from build123d import *

# Parameters (mm, degrees)
SKETCH1_W           = 16
SKETCH1_H           = 9
BOSS_EXTRUDE1_DEPTH = 3


with BuildPart() as part:
    # Sketch1 → Boss-Extrude1 (new body)
    with BuildSketch(Plane(origin=(0, 0, 0), x_dir=(0, 0, -1), z_dir=(1, 0, 0))):
        Polygon((10, 153.005875518), (20, 153.005875518), (20, 150.005875518), (30, 150.005875518), (30, 153.005875518), (40, 153.005875518), (40, 150.005875518), (50, 150.005875518), (50, 153.005875518), (60, 153.005875518), (60, 150.005875518), (70, 150.005875518), (70, 140), (73, 140), (73, 130), (70, 130), (70, 120), (73, 120), (73, 110), (70, 110), (70, 100), (73, 100), (73, 90), (70, 90), (70, 80), (73, 80), (73, 70), (70, 70), (70, 60), (73, 60), (73, 50), (70, 50), (70, 40), (73, 40), (73, 30), (70, 30), (70, 20), (73, 20), (73, 10), (70, 10), (70, 0), (60, 0), (60, -3), (50, -3), (50, 0), (40, 0), (40, -3), (30, -3), (30, 0), (20, 0), (20, -3), (10, -3), (10, 0), (0, 0), (0, 10), (-3, 10), (-3, 20), (0, 20), (0, 30), (-3, 30), (-3, 40), (0, 40), (0, 50), (-3, 50), (-3, 60), (0, 60), (0, 70), (-3, 70), (-3, 80), (0, 80), (0, 90), (-3, 90), (-3, 100), (0, 100), (0, 110), (-3, 110), (-3, 120), (0, 120), (0, 130), (-3, 130), (-3, 140), (0, 140), (0, 150.005875518), (10, 150.005875518), align=None)
        with Locations((33.90899457, 144.39356925)):
            Rectangle(SKETCH1_W, SKETCH1_H, mode=Mode.SUBTRACT)
    extrude(amount=BOSS_EXTRUDE1_DEPTH)


solid = part.part
Check sheet for the modelled part. Datum: model origin and axes. Units: mm. A direction names the side the tool comes from. Round coordinates to 2 decimals unless told otherwise and drop trailing zeros. Loops run counter-clockwise (first coordinate to the right, second up) from the corner with the lowest first, then second, coordinate; pieces in that order, holes last.
1. Sectioned sample at C-C on z = -62. Record the boundary of the cut face in (x, y).
2. Set-up check for faces 5 (the flat face through (1, 139.894, -34)), 6 (the flat face through (1, 140, 2)), 7 (the flat face through (1, 130, 1)), 8 (the flat face through (1, 150.006, -45)), 9 (the flat face through (1, 130, -72)): record each of +Z, -Z, +X, -X, +Y, -Y from which the full face is reachable in a straight line by a thin tool's end or side.
3. Scan lines: probe 1 along Y at (x, z) = (1.95, -32.5); probe 2 along Y at (x, z) = (2, -41); probe 3 along Z at (x, y) = (2.4, 47). Record each from-to range of solid material in increasing order.
4. Gauge pin test, flat ends, axial feed: pin 1 Ø1.5 at (x, y) = (1, 65.5) entering from -Z; pin 2 Ø0.9 at (x, z) = (1, -4.5) entering from -Y; pin 3 Ø1.5 at (x, z) = (1, -71) entering from +Y. Record the tip position at first contact, or that the pin passes through.
5. Mould release check, pull along Y, two halves, no side actions. Record for faces 1 (the flat face through (1, 90, 1)), 2 (the flat face through (1, -1, -20)), 3 (the flat face through (1, 10, -72)), 4 (the flat face through (1, 105, 0)): released by +Y, released by -Y, zero draft, split by the parting line, or undercut.
6. Sectioned sample at B-B on y = 123. Record the boundary of the cut face in (x, z), and give its area (3 significant figures).
7. Sectioned sample at A-A on z = -35. Record the boundary of the cut face in (x, y), and give its area (3 significant figures).
Recorded:
1. outline: (0, 0) - (3, 0) - (3, 150.01) - (0, 150.01) - close
2. face 5: +X, -X
2. face 6: +Z, +X, -X, +Y
2. face 7: +Z, +X, -X
2. face 8: +X, -X, +Y
2. face 9: -Z, +X, -X
3. probe 1: y = -3 to 139.89, 148.89 to 153.01
3. probe 2: y = 0 to 139.89, 148.89 to 150.01
3. probe 3: z = -70 to 0
4. pin 1: stops at z = -70
4. pin 2: stops at y = 0
4. pin 3: stops at y = 140
5. face 1: undercut
5. face 2: zero draft
5. face 3: released by -Y
5. face 4: undercut
6. outline: (0, -70) - (3, -70) - (3, 0) - (0, 0) - close
6. area: 210 mm2
7. outline: (0, -3) - (3, -3) - (3, 139.89) - (0, 139.89) - close; (0, 148.89) - (3, 148.89) - (3, 153.01) - (0, 153.01) - close
7. area: 441 mm2
